Part print with two shaded views. Sizes in mm from the minimum x, y, z corner. A direction names the side the tool comes from. Give positions to 0.01 mm unless a question says otherwise; leave off trailing zeros. Write each loop counter-clockwise with the first axis right and the second up, starting at its lowest first coordinate (ties: lowest second). Pieces come first, ordered by that corner, then holes. Notation, with made-up numbers: M 4,7 L 62,7 A37 cw 62,43 Z; hole C 74.5,-33 d11. An arc over 180 degrees is marked long. One line per item, written item: value. Start each with the question number.
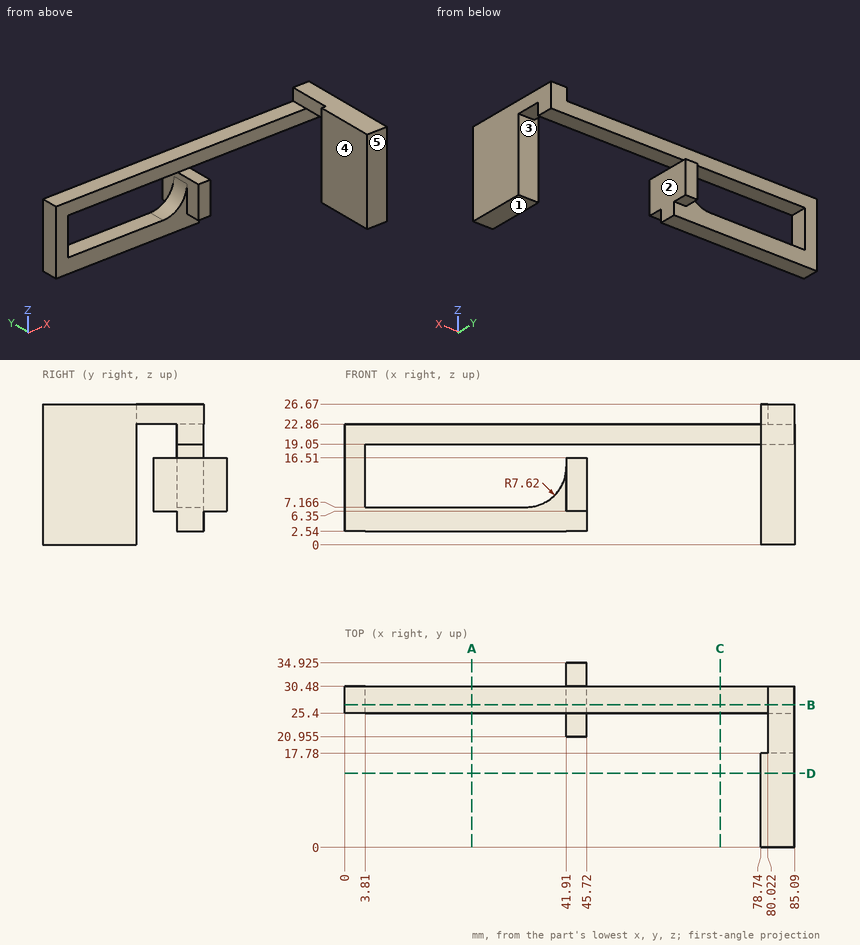
1) Band-saw the part on C-C (x = 71). List the corners of the cut face in (y, z).
2) Probe line 1 along X through (y, z) = (5.5, 1.75); line 2 along Y through (x, z) = (79, 25); line 3 along Z through (x, y) = (44.5, 25). List the from-to ranges inside material, lowest first. Write a range as from..to.
3) Band-saw the part on B-B (y = 27). List the corners of the cut face in (x, z).
4) Drop flat-ended pins along their axis: P1, Ø5, axis at y = 10.5, z = 3, coming from the -X side; P2, Ø1.1, axis at x = 43.5, z = 13.5, coming from the -Y side (3 decimals); P3, Ø4, axis at x = 44.5, y = 23.5, coming from the -Z side; P4, Ø12, axis at x = 30, y = 17.5, coming from the -Z side. Give the stop position or say it passes through.
5) Band-saw the part on D-D (y = 14). List the corners of the cut face in (x, z), then the cut area to 3 significant figures.
6) Mould opens along Y. For the marked faces 3, 4 and 5 say: released by +Y, released by -Y, zero draft, split by the parting line, or undercut.
7) Band-saw the part on A-A (x = 24). List the corners of the cut face in (y, z).
8) Tool access for the marked faces 1 and 2: list every direction of +Z, -Z, +X, -X, +Y, -Y with a clear straight run to the whole face (end or side of a thin tool).
Model answer:
1. outline: M 25.4,19.05 L 30.48,19.05 L 30.48,22.86 L 25.4,22.86 Z
2. line 1: x = 78.74..85.09
2. line 2: y = 0..17.78
2. line 3: z = 6.35..16.51
3. outline: M 0,2.54 L 45.72,2.54 L 45.72,16.51 L 41.91,16.51 L 41.91,14.79 A7.62 cw 34.29,7.17 L 3.81,7.17 L 3.81,19.05 L 85.09,19.05 L 85.09,26.67 L 80.02,26.67 L 80.02,22.86 L 0,22.86 Z
4. P1: stops at x = 78.74
4. P2: stops at y = 20.955
4. P3: stops at z = 2.54
4. P4: passes through
5. outline: M 78.74,0 L 85.09,0 L 85.09,26.67 L 78.74,26.67 Z
5. area: 169 mm²
6. face 3: undercut
6. face 4: zero draft
6. face 5: released by -Y
7. outline: M 25.4,2.54 L 30.48,2.54 L 30.48,7.17 L 25.4,7.17 Z; M 25.4,19.05 L 30.48,19.05 L 30.48,22.86 L 25.4,22.86 Z
8. face 1: -Z, +X, -X, +Y, -Y
8. face 2: -Z, +X, +Y, -Y
